Verification items for this drawing (mm, ordinates from the low corner). A direction names the side the tool comes from. Coordinates: 2 decimals unless noted, no trailing zeros. Loops run counter-clockwise (first coordinate to the right, second up) from the corner with the lowest first, then second, coordinate; pieces in that order, holes last. Notation, with made-up numbers: (17, 5.25) - (53, 5.25) arc R27 cw to (53, 33.25) - close; hole circle Ø11 at (-38.5, 28). An arc over 180 degrees is marked (long way). One line per item, written item: value. Start each with the question number.
(1) Section check B-B (x = 106.5). Record the boundary of the cut face in (y, z).
(2) Set-up check for the marked faces 1, 2 and 3: record each of +Z, -Z, +X, -X, +Y, -Y from which the full face is reachable in a straight line by a thin tool's end or side.
(3) Thickness scan on probe 1 along X at (y, z) = (45, 6.5); probe 2 along Z at (x, y) = (35, 8); probe 3 along X at (y, z) = (24.5, 14) (1 decimal). Record the ranges inside material, lowest first. Write a range as [from, to].
(4) Section check C-C (x = 13). Record the boundary of the cut face in (y, z), plus the area to 3 significant figures.
(5) Gauge pin test, flat ends, axial feed: P1, Ø10, axis at x = 6.5, y = 87, coming from the +Z side; P2, Ø10, axis at x = 118.5, y = 25.5, coming from the +Z side; P3, Ø3, axis at x = 114, z = 8.5, coming from the +Y side. Record the tip position at first contact, or that the pin passes through.
(6) Section check A-A (z = 5). Record the boundary of the cut face in (x, y) (1 decimal).
(7) Section check D-D (z = 33.5). Record the boundary of the cut face in (x, y), plus the area to 3 significant figures.
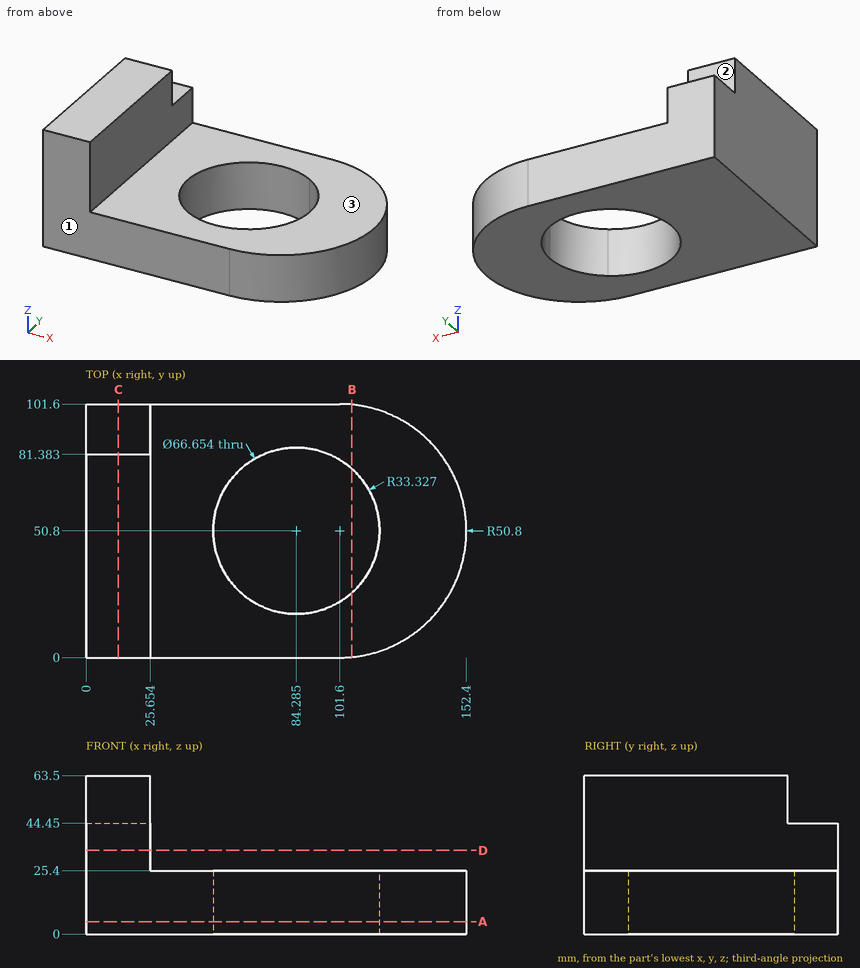
Responses:
1. outline: (0.24, 0) - (25.96, 0) - (25.96, 25.4) - (0.24, 25.4) - close; (75.64, 0) - (101.36, 0) - (101.36, 25.4) - (75.64, 25.4) - close
2. face 1: +Z, -Z, +X, -X, -Y
2. face 2: +Z, +X, -X, +Y
2. face 3: +Z, +X, +Y, -Y
3. probe 1: x = [0, 51.47], [117.1, 152.07]
3. probe 2: z = [0, 25.4]
3. probe 3: x = [0, 63.8], [104.8, 145.1]
4. outline: (0, 0) - (101.6, 0) - (101.6, 44.45) - (81.38, 44.45) - (81.38, 63.5) - (0, 63.5) - close
4. area: 6,070 mm²
5. P1: stops at z = 44.45
5. P2: stops at z = 25.4
5. P3: stops at y = 100.42
6. outline: (0, 0) - (101.6, 0) arc R50.8 ccw to (101.6, 101.6) - (0, 101.6) - close; hole (101.6, 22.3) arc R33.3 ccw to (117.6, 50.8) arc R33.3 ccw to (101.6, 79.3) arc R33.3 ccw (long way) to start
7. outline: (0, 0) - (25.65, 0) - (25.65, 101.6) - (0, 101.6) - close
7. area: 2,610 mm²
